from build123d import *

# Parameters (mm, degrees)
F0_W     = 95.8622172475
F0_H     = 56.4189068973
F1_DEPTH = 25.4
F2_W     = 95.8622172475
F2_H     = 7.8636966646
F2_H_2   = 7.364413701
F3_DEPTH = 6.604
F4_W     = 41.1907965317
F4_H     = 22.9055710793
F5_DEPTH = 42.926
F6_R     = 9.155401704
F6_R_2   = 8.8261485634
F7_DEPTH = 92.964


with BuildPart() as f1:
    # F0 (on Top) → F1 (new body)
    with BuildSketch(Plane.XY):
        with Locations((9.2367231846, -8.8622625917)):
            Rectangle(F0_W, F0_H)
    extrude(amount=F1_DEPTH)

    # F2 (on face) → F3 (cut)
    with BuildSketch(Plane.XY.offset(25.4)):
        with Locations((9.2367231846, -33.1398677081)):
            Rectangle(F2_W, F2_H)
        with Locations((9.2367231846, 15.6649840064)):
            Rectangle(F2_W, F2_H_2)
    extrude(amount=-F3_DEPTH, mode=Mode.SUBTRACT)

    # F4 (on face) → F5 (join)
    with BuildSketch(Plane(origin=(-38.6943854392, 0, 0), x_dir=(0, -1, 0), z_dir=(-1, 0, 0))):
        with Locations((8.6126211099, 36.8527855396)):
            Rectangle(F4_W, F4_H)
    extrude(amount=-F5_DEPTH)

    # F6 (on Top) → F7 (cut)
    with BuildSketch(Plane.XY):
        with Locations((-17.3500627279, -9.2367241159)):
            Circle(F6_R)
        with Locations((30.5810458958, -9.2367241159)):
            Circle(F6_R_2)
    extrude(amount=F7_DEPTH, mode=Mode.SUBTRACT)


solid = f1.part
The listing builds one solid part. Answer for the finished solid, in the listing's coordinates (mm). A direction names the side the tool comes from. Give positions to 0.01 mm unless a question says otherwise; leave off trailing zeros. Order: outer loops, then holes, each group sorted by start corner. A loop starts at its lowest first (then second) coordinate and runs counter-clockwise, first axis right, second up. Notation, with made-up numbers: (57, 30) -> (75, 30) arc R24 ccw to (75, 44) -> close; hole circle Ø11 at (13, 43.5). An arc over 180 degrees is marked (long way). Put each result on its own line as item: value.
Item 1: For a pull along X with two mould halves and no side action, classify faces 1 (the face through (28.668, -17.853, 12.522)), 2 (the face through (9, -8, 0)), 3 (the face through (57.168, -9, 13)) as released by +X, released by -X, zero draft, split by the parting line, or undercut.
Established:
face 1: undercut
face 2: zero draft
face 3: released by +X
Item 2: Straight lines are drawn through the part: line 1 (Y direction, x = -17.5, z = 3); line 2 (X direction, y = -4, z = 6); line 3 (Z direction, x = 22, y = -13.5). For each, find the intervals that lie inside material, in ascending order.
Established:
line 1: y = -37.07 to -18.39, -0.08 to 19.35
line 2: x = -38.69 to -24.86, -9.84 to 23.48, 37.69 to 57.17
line 3: z = 0 to 25.4
Item 3: A cutting plane is placed at A-A on y = -15. Give the vertices of the cut face in (x, z), plus the area to 3 significant figures.
Established:
outline: (-38.69, 0) -> (-24.46, 0) -> (-24.46, 48.31) -> (-38.69, 48.31) -> close; (-10.24, 0) -> (23.9, 0) -> (23.9, 25.4) -> (4.23, 25.4) -> (4.23, 48.31) -> (-10.24, 48.31) -> close; (37.27, 0) -> (57.17, 0) -> (57.17, 25.4) -> (37.27, 25.4) -> close
area: 2,390 mm^2
Item 4: A cutting plane is placed at C-C on x = 33.5. Give the vertices of the cut face in (y, z), plus the area to 3 significant figures.
Established:
outline: (-37.07, 0) -> (-17.57, 0) -> (-17.57, 25.4) -> (-29.21, 25.4) -> (-29.21, 18.8) -> (-37.07, 18.8) -> close; (-0.91, 0) -> (19.35, 0) -> (19.35, 18.8) -> (11.98, 18.8) -> (11.98, 25.4) -> (-0.91, 25.4) -> close
area: 909 mm^2
Item 5: A cutting plane is placed at B-B on x = -29.5. Give the vertices of the cut face in (y, z), plus the area to 3 significant figures.
Established:
outline: (-37.07, 0) -> (19.35, 0) -> (19.35, 18.8) -> (11.98, 18.8) -> (11.98, 48.31) -> (-29.21, 48.31) -> (-29.21, 18.8) -> (-37.07, 18.8) -> close
area: 2,280 mm^2
Item 6: For faces 4 (the face through (4.232, -8, 37)), 5 (the face through (9, -33, 18.796)), 6 (the face through (9, 16, 18.796)), determine the directions among +Z, -Z, +X, -X, +Y, -Y from which every point of the face is accessible in a straight line to the end or side of a thin tool.
Established:
face 4: +Z, +X, +Y, -Y
face 5: +Z, +X, -X, -Y
face 6: +Z, +X, -X, +Y
Item 7: A cutting plane is placed at D-D on z = 26.5. Give the vertices of the cut face in (x, y).
Established:
outline: (-38.69, -29.21) -> (4.23, -29.21) -> (4.23, 11.98) -> (-38.69, 11.98) -> close; hole circle Ø18.31 at (-17.35, -9.24)
Item 8: Given P1, Ø8, axis at x = -12, y = 14.5, coming from the +Z side; P2, Ø4, axis at x = 8, y = -32, coming from the +Z side; P3, Ø12.5, axis at x = 26.5, y = -5, coming from the +Z side; P4, Ø9, axis at x = -2.5, z = 39.5, coming from the -Y side, each flat-ended and moving along its own axis, determine where each tip first touches the part or whether it passes through.
Established:
P1: stops at z = 48.31
P2: stops at z = 18.8
P3: stops at z = 25.4
P4: stops at y = -29.21
